Could you check a few things on this model? Use its own coordinates, in mm. A direction names the side the tool comes from. Give positions to 0.01 mm unless a question says otherwise; leave off trailing zeros. Write each loop counter-clockwise with the first axis right and the second up, starting at its lowest first coordinate (ties: lowest second). Pieces come first, ordered by that corner, then holes. Notation, with made-up numbers: (30, -38.75) - (43, -38.75) arc R14 cw to (43, -19.75) - close; hole circle Ø9 at (-32, 2). An arc over 180 degrees is marked (long way). Use one line per item in the form item = value.
Autodesk Inventor part; units mm, degrees
ref_plane "YZ Plane" through (0, 0, 0) normal (1, 0, 0) x (0, 1, 0)
ref_plane "XZ Plane" through (0, 0, 0) normal (0, 1, 0) x (-1, 0, 0)
ref_plane "XY Plane" through (0, 0, 0) normal (0, 0, 1) x (1, 0, 0)
sketch "Sketch1" plane through (0, 0, 0) normal (0, 1, 0) x (-1, 0, 0)
  circle A0 centre (0, 0) radius 4
  circle A1 centre (0, 0) radius 16
  dimension "d0" = 8
  dimension "d1" = 32
extrude "Extrusion1" add sketch "Sketch1" along normal blind 5
sketch "Sketch2" plane through (0, 5, 0) normal (0, 1, 0) x (1, 0, 0)
  circle A0 centre (0, 0) radius 4
  circle A1 centre (0, 0) radius 7.5
  dimension "d4" = 15
extrude "Extrusion2" add sketch "Sketch2" along normal blind 19
sketch "Sketch3" plane through (0, 0, 0) normal (0, -1, 0) x (1, 0, 0)
  point P0 (0, 0)
sketch "Sketch4" plane through (0, 0, 0) normal (0, -1, 0) x (1, 0, 0)
  circle A0 centre (0, 12) radius 1.75
  point P0 (0, 0)
  dimension "d8" = 3.5
extrude "Extrusion3" cut sketch "Sketch4" against normal blind 19
pattern_circular "Circular Pattern1" count 4 over 360 about axis through (0, -10, 0) along (0, 1, 0) of "Extrusion3"
properties part number "Soporte Eje"
1. Imagine slicing it at D-D, the plane y = 20.5. List the corners of the cut face in (x, z) for me.
Response values:
outline = circle Ø15 at (0, 0); hole circle Ø8 at (0, 0)
2. Imagine slicing it at C-C, the plane x = -12. List the corners of the cut face in (y, z) for me, and give its area (3 significant figures).
Response values:
outline = (0, -10.58) - (5, -10.58) - (5, -1.75) - (0, -1.75) - close; (0, 1.75) - (5, 1.75) - (5, 10.58) - (0, 10.58) - close
area = 88.3 mm²
3. Imagine slicing it at B-B, the plane z = 12. List the corners of the cut face in (x, y) for me.
Response values:
outline = (-10.58, 0) - (-1.75, 0) - (-1.75, 5) - (-10.58, 5) - close; (1.75, 0) - (10.58, 0) - (10.58, 5) - (1.75, 5) - close
4. For pin 1 (6.5 mm diameter, centred on x = 0, z = 0, fed in from +Y); pin 2 (12 mm diameter, centred on y = 4.5, z = 11, fed in from -X); pin 3 (4 mm diameter, centred on y = 14, z = -1, fed in from -X); pin 4 (1 mm diameter, centred on x = 5.5, y = 8, fed in from +Z), each with a flat end and sliding along its axis, tell me the tip position at first contact or that it passes through.
Response values:
pin_1 = through
pin_2 = -15.2
pin_3 = -7.5
pin_4 = 5.59
5. If I drill on line 1 (Z direction, x = 0, y = 1.35); line 2 (Z direction, x = 0, y = 5.5); line 3 (X direction, y = 2.5, z = 1), over which ranges is the centre line in solid material (lowest first)? Write a range as from..to.
Response values:
line_1 = -16..-13.75, -10.25..-4, 4..10.25, 13.75..16
line_2 = -7.5..-4, 4..7.5
line_3 = -15.97..-13.44, -10.56..-3.87, 3.87..10.56, 13.44..15.97
6. If we mould it in two halves opening along Z, with no side actions, what happens to faces 1 (the face through (-13.735, 2.465, -0.228)), 2 (the face through (3.47, 2.46, 15.62)), 3 (the face through (-3, 0, -3))? For each: pulls with the +Z half, pulls with the -Z half, needs draft (parallel to the pull), parting line crosses it, or undercut.
Response values:
face_1 = undercut
face_2 = parting line crosses it
face_3 = needs draft
7. Which directions (+Z, -Z, +X, -X, +Y, -Y) give clear straight access to the entire face, cutting with the end or side of a thin tool? Please do faces 4 (the face through (13.735, 2.465, 0.228)), 5 (the face through (-7.493, 14.367, 0.33)).
Response values:
face_4 = +Y, -Y
face_5 = +Y
